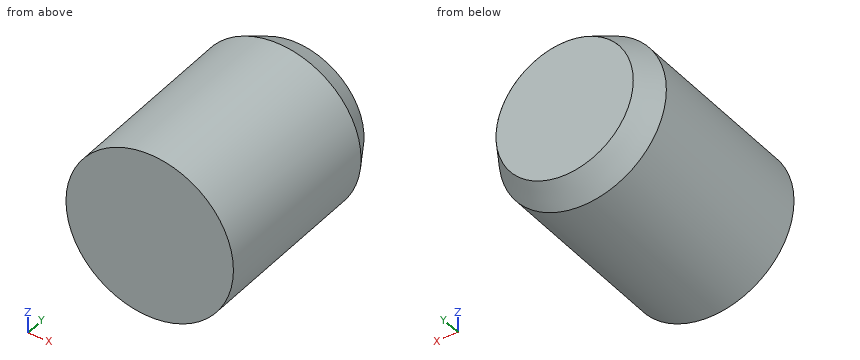
Autodesk Inventor part; units mm, degrees
ref_plane "YZ Plane" through (0, 0, 0) normal (1, 0, 0) x (0, 1, 0)
ref_plane "XZ Plane" through (0, 0, 0) normal (0, 1, 0) x (-1, 0, 0)
ref_plane "XY Plane" through (0, 0, 0) normal (0, 0, 1) x (1, 0, 0)
sketch "Sketch1" plane through (0, 0, 0) normal (0, 1, 0) x (-1, 0, 0)
  circle A0 centre (0, 0) radius 5.55
  dimension "d0" = 11.1
extrude "Extrusion1" add sketch "Sketch1" along normal blind 14
sketch "Sketch2" plane through (0, 14, 0) normal (0, 1, 0) x (1, 0, 0)
  circle A0 centre (0, 0) radius 4.55
  circle A1 centre (0, 0) radius 5.55
  dimension "d3" = 1
extrude "Extrusion2" cut sketch "Sketch2" against normal blind 12 contours A0
chamfer "Chamfer1" distance 1 angle 60 1 edges at (5.55, 14, 0) measured on face at (-5.1629, 14, -0.4427)
properties part number "Plug_3DPrint"
Model file for the job. Use its own axes, mm. Coordinates: 2 decimals unless noted, no trailing zeros. Order: outer loops, then holes, each group sorted by start corner. A loop starts at its lowest first (then second) coordinate and runs counter-clockwise, first axis right, second up. Notation, with made-up numbers: (-17.5, -28.75) -> (10.5, -28.75) arc R21 ccw to (10.5, 10.25) -> close; hole circle Ø7 at (27.5, -39). An arc over 180 degrees is marked (long way). Answer as a JSON object with one key per item and string values. Group by question number.
1) Flat gauge pins, fed straight in: pin 1 (2 mm diameter, centred on y = 12.5, z = 4.5, fed in from +X); pin 2 (5 mm diameter, centred on x = -0.5, z = 0.5, fed in from +Y); pin 3 (1 mm diameter, centred on x = 2, y = 2, fed in from -Z). Where does each tip first touch, or does it go through?
2) Drill centre lines: L1, parallel to Z at x = 0, y = 10.5; L2, parallel to Y at x = 0.25, z = -3; L3, parallel to X at y = 10.5, z = -0.75. Where is each one in solid material? Low to high.
3) Cut at C-C, the plane y = 4.75. Write the cut outline in (x, z), then the cut area to 3 significant figures.
Check values:
{
 "1": {"pin 1": "stops at x = 4.28", "pin 2": "stops at y = 2", "pin 3": "stops at z = -5.34"},
 "2": {"L1": "z = -5.55 to -4.55, 4.55 to 5.55", "L2": "y = 0 to 2", "L3": "x = -5.5 to -4.49, 4.49 to 5.5"},
 "3": {"outline": "circle Ø11.1 at (0, 0); hole circle Ø9.1 at (0, 0)", "area": "31.7 mm²"}
}
